```python
from build123d import *

# Parameters (mm, degrees)
SKETCH1_W             = 40
SKETCH1_H             = 51.5
BOSS_EXTRUDE1_DEPTH   = 18
SKETCH3_R             = 1.6
CUT_EXTRUDE1_DEPTH    = 19
SKETCH4_R             = 3.5
CUT_EXTRUDE2_DEPTH    = 18
CUT_EXTRUDE3_DEPTH    = 8
SKETCH6_R             = 9
CUT_EXTRUDE4_DEPTH    = 8
SKETCH7_R             = 7
CUT_EXTRUDE5_DEPTH    = 2.8
SKETCH8_R             = 6
CUT_EXTRUDE6_DEPTH    = 3.8
SKETCH9_R             = 5
CUT_EXTRUDE7_DEPTH    = 8
M3X0_5_TAPPED_HOLE1_D = 2.5
CUT_EXTRUDE8_DEPTH    = 2
CUT_EXTRUDE9_DEPTH    = 1
CHAMFER1_SIZE         = 0.8
SKETCH14_W            = 1
SKETCH14_H            = 6.5
CUT_EXTRUDE10_DEPTH   = 7


with BuildPart() as part:
    # Sketch1 → Boss-Extrude1 (new body)
    with BuildSketch(Plane.XY):
        Rectangle(SKETCH1_W, SKETCH1_H)
    extrude(amount=BOSS_EXTRUDE1_DEPTH)

    # Sketch3 → Cut-Extrude1 (cut, through all)
    with BuildSketch(Plane.XY.offset(18)):
        with Locations((-15, 21.5)):
            Circle(SKETCH3_R)
        with Locations((-15, -21.5)):
            Circle(SKETCH3_R)
        with Locations((15, 21.5)):
            Circle(SKETCH3_R)
        with Locations((15, -21.5)):
            Circle(SKETCH3_R)
    extrude(amount=-CUT_EXTRUDE1_DEPTH, mode=Mode.SUBTRACT)

    # Sketch4 → Cut-Extrude2 (cut)
    with BuildSketch(Plane.XY.offset(18)):
        with Locations((0, -14.25)):
            Circle(SKETCH4_R)
    extrude(amount=-CUT_EXTRUDE2_DEPTH, mode=Mode.SUBTRACT)

    # Sketch5 → Cut-Extrude3 (cut)
    with BuildSketch(Plane.XY.offset(18)):
        with BuildLine():
            Line((-17, 17.872848693), (-17, -17.872848693))
            ThreePointArc((-17, -17.872848693), (-17.124132538, -18.49783351), (-17.477686074, -19.027941805))
            ThreePointArc((-17.477686074, -19.027941805), (-17.229095042, -24.198357888), (-12.104699799, -23.466529111))
            ThreePointArc((-12.104699799, -23.466529111), (-11.517289712, -22.940191537), (-10.751842764, -22.75))
            Line((-10.751842764, -22.75), (-9.2376, -22.75))
            ThreePointArc((-9.2376, -22.75), (-8.237593216, -22.482046891), (-7.50554136, -21.749986433))
            Line((-7.50554136, -21.749986433), (-4.85642932, -17.161506784))
            ThreePointArc((-4.85642932, -17.161506784), (-4.082002001, -16.665704301), (-3.230119897, -17.011904614))
            ThreePointArc((-3.230119897, -17.011904614), (-3.134851007, -17.11961684), (-3.035950666, -17.224004614))
            ThreePointArc((-3.035950666, -17.224004614), (-2.824243732, -17.545979208), (-2.75, -17.9241))
            Line((-2.75, -17.9241), (-2.75, -20.75))
            ThreePointArc((-2.75, -20.75), (-2.164213562, -22.164213562), (-0.75, -22.75))
            Line((-0.75, -22.75), (10.751842764, -22.75))
            ThreePointArc((10.751842764, -22.75), (11.517289712, -22.940191537), (12.104699799, -23.466529111))
            ThreePointArc((12.104699799, -23.466529111), (17.229095042, -24.198357888), (17.477686074, -19.027941805))
            ThreePointArc((17.477686074, -19.027941805), (17.124132538, -18.49783351), (17, -17.872848693))
            Line((17, -17.872848693), (17, 17.872848693))
            ThreePointArc((17, 17.872848693), (17.124132538, 18.49783351), (17.477686074, 19.027941805))
            ThreePointArc((17.477686074, 19.027941805), (17.229095042, 24.198357888), (12.104699799, 23.466529111))
            ThreePointArc((12.104699799, 23.466529111), (11.517289712, 22.940191537), (10.751842764, 22.75))
            Line((10.751842764, 22.75), (-10.751842764, 22.75))
            ThreePointArc((-10.751842764, 22.75), (-11.517289712, 22.940191537), (-12.104699799, 23.466529111))
            ThreePointArc((-12.104699799, 23.466529111), (-17.229095042, 24.198357888), (-17.477686074, 19.027941805))
            ThreePointArc((-17.477686074, 19.027941805), (-17.124132538, 18.49783351), (-17, 17.872848693))
        make_face()
    extrude(amount=-CUT_EXTRUDE3_DEPTH, mode=Mode.SUBTRACT)

    # Sketch6 → Cut-Extrude4 (cut)
    with BuildSketch(Plane(origin=(0, 0, 0), x_dir=(-1, 0, 0), z_dir=(0, 0, -1))):
        with BuildLine():
            Line((-20, 10.5), (-15.5, 10.5))
            ThreePointArc((-15.5, 10.5), (-12.25, 7.25), (-15.5, 4))
            Line((-15.5, 4), (-20, 4))
            Line((-20, 4), (-20, -25.75))
            Line((-20, -25.75), (20, -25.75))
            Line((20, -25.75), (20, 4))
            Line((20, 4), (15.5, 4))
            ThreePointArc((15.5, 4), (12.25, 7.25), (15.5, 10.5))
            Line((15.5, 10.5), (20, 10.5))
            Line((20, 10.5), (20, 25.75))
            Line((20, 25.75), (-20, 25.75))
            Line((-20, 25.75), (-20, 10.5))
        make_face()
        with Locations((0, -14.25)):
            Circle(SKETCH6_R, mode=Mode.SUBTRACT)
    extrude(amount=-CUT_EXTRUDE4_DEPTH, mode=Mode.SUBTRACT)

    # Sketch7 → Cut-Extrude5 (cut)
    with BuildSketch(Plane(origin=(0, 0, 0), x_dir=(-1, 0, 0), z_dir=(0, 0, -1))):
        with Locations((0, -14.25)):
            Circle(SKETCH7_R)
    extrude(amount=-CUT_EXTRUDE5_DEPTH, mode=Mode.SUBTRACT)

    # Sketch8 → Cut-Extrude6 (cut)
    with BuildSketch(Plane(origin=(0, 0, 0), x_dir=(-1, 0, 0), z_dir=(0, 0, -1))):
        with Locations((0, -14.25)):
            Circle(SKETCH8_R)
    extrude(amount=-CUT_EXTRUDE6_DEPTH, mode=Mode.SUBTRACT)

    # Sketch9 → Cut-Extrude7 (cut)
    with BuildSketch(Plane(origin=(0, 0, 0), x_dir=(-1, 0, 0), z_dir=(0, 0, -1))):
        with Locations((0, -14.25)):
            Circle(SKETCH9_R)
    extrude(amount=-CUT_EXTRUDE7_DEPTH, mode=Mode.SUBTRACT)

    # M3x0.5 Tapped Hole1 (through all)
    with Locations(Plane(origin=(0, 0, 0), x_dir=(-1, 0, 0), z_dir=(0, 0, -1))):
        with Locations((-15.5, 7.25), (15.5, 7.25)):
            Hole(M3X0_5_TAPPED_HOLE1_D / 2)

    # Sketch12 → Cut-Extrude8 (cut)
    with BuildSketch(Plane(origin=(0, 0, 8), x_dir=(-1, 0, 0), z_dir=(0, 0, -1))):
        with BuildLine():
            Line((-8, 17.401970252), (-8, 25.75))
            Line((-8, 25.75), (8, 25.75))
            Line((8, 25.75), (8, 17.401970252))
            ThreePointArc((8, 17.401970252), (8.155139905, 16.629641806), (8.596491228, 15.977132322))
            ThreePointArc((8.596491228, 15.977132322), (0, -5), (-8.596491228, 15.977132322))
            ThreePointArc((-8.596491228, 15.977132322), (-8.155139905, 16.629641806), (-8, 17.401970252))
        make_face()
    extrude(amount=-CUT_EXTRUDE8_DEPTH, mode=Mode.SUBTRACT)

    # Sketch13 → Cut-Extrude9 (cut)
    with BuildSketch(Plane(origin=(0, 0, 0), x_dir=(-1, 0, 0), z_dir=(0, 0, -1))):
        with BuildLine():
            Line((-20, 10.5), (-20, 4))
            Line((-20, 4), (-15.5, 4))
            ThreePointArc((-15.5, 4), (-12.25, 7.25), (-15.5, 10.5))
            Line((-15.5, 10.5), (-20, 10.5))
        make_face()
        with BuildLine():
            Line((20, 4), (20, 10.5))
            Line((20, 10.5), (15.5, 10.5))
            ThreePointArc((15.5, 10.5), (12.25, 7.25), (15.5, 4))
            Line((15.5, 4), (20, 4))
        make_face()
    extrude(amount=-CUT_EXTRUDE9_DEPTH, mode=Mode.SUBTRACT)

    # Chamfer1
    chamfer1_edges = [part.edges().sort_by_distance(p)[0] for p in [
        (20, -25.75, 13),
        (-20, -25.75, 13),
        (-20, 25.75, 13),
        (20, 25.75, 13),
    ]]
    chamfer(chamfer1_edges, length=CHAMFER1_SIZE)

    # Sketch14 → Cut-Extrude10 (cut)
    with BuildSketch(Plane(origin=(0, 0, 1), x_dir=(-1, 0, 0), z_dir=(0, 0, -1))):
        with Locations((-19.5, 7.25)):
            Rectangle(SKETCH14_W, SKETCH14_H)
        with Locations((19.5, 7.25)):
            Rectangle(SKETCH14_W, SKETCH14_H)
    extrude(amount=-CUT_EXTRUDE10_DEPTH, mode=Mode.SUBTRACT)


solid = part.part
```
Model file for the job. Use its own axes, mm. A direction names the side the tool comes from. Round coordinates to 2 decimals unless told otherwise and drop trailing zeros. Order: outer loops, then holes, each group sorted by start corner. A loop starts at its lowest first (then second) coordinate and runs counter-clockwise, first axis right, second up. Notation, with made-up numbers: (-1.5, 9) -> (40.5, 9) arc R20 ccw to (40.5, 14) -> close; hole circle Ø4 at (9.5, 82.25). An arc over 180 degrees is marked (long way). Use one line per item in the form item = value.
Item 1: Drill centre lines: line 1 (X direction, y = -10.5, z = 14); line 2 (Y direction, x = 8, z = 14.5); line 3 (Y direction, x = -15, z = 9.4). Where is each one in solid material? Low to high.
Returned:
line_1 = -20 to -17, 17 to 20
line_2 = -25.75 to -22.75, 22.75 to 25.75
line_3 = -25.75 to -23.1, -19.9 to 6.1, 8.4 to 19.9, 23.1 to 25.75
Item 2: Cut at B-B, the plane z = 4.75. Write the cut outline in (x, y), and give its area (3 significant figures).
Returned:
outline = (-19, 4) -> (-15.5, 4) arc R3.25 ccw to (-15.5, 10.5) -> (-19, 10.5) -> close; circle Ø18 at (0, -14.25); (15.5, 4) -> (19, 4) -> (19, 10.5) -> (15.5, 10.5) arc R3.25 ccw to start; hole circle Ø2.5 at (-15.5, 7.25); hole circle Ø10 at (0, -14.25); hole circle Ø2.5 at (15.5, 7.25)
area = 245 mm^2
Item 3: Cut at C-C, the plane x = 0. Give the number of separate pieces and of enclosed holes in the cut face, and give its area (3 significant figures).
Returned:
separate_pieces = 3
enclosed_holes = 0
area = 126 mm^2
Item 4: Flat gauge pins, fed straight in: pin 1 Ø3.5 at (x, y) = (15, 21.5) entering from -Z; pin 2 Ø2 at (y, z) = (10.5, 4.5) entering from +X; pin 3 Ø2 at (x, y) = (15.5, 8.5) entering from -Z. Where does each tip first touch, or does it go through?
Returned:
pin_1 = 8
pin_2 = 19
pin_3 = 1
Item 5: Tool access for faces 1 (the face through (-8.15, 16.64, 8.99)), 2 (the face through (-17, 4, 4)), 3 (the face through (17.166, -24.25, 14.056)), 4 (the face through (-6, -12, 2.8)): list every direction of +Z, -Z, +X, -X, +Y, -Y with a clear straight run to the whole face (end or side of a thin tool).
Returned:
face_1 = +Z, -Z
face_2 = -Z, +X, -X, -Y
face_3 = +Z
face_4 = -Z
Item 6: Pull direction X, two halves, no side cores. Call faces 5 (the face through (20, 0, 13)), 6 (the face through (0, -25.75, 13)), 7 (the face through (-6.2, -19.49, 14.06)), 8 (the face through (-19, 7, 4)): released by +X, released by -X, zero draft, split by the parting line, or undercut.
Returned:
face_5 = released by +X
face_6 = zero draft
face_7 = undercut
face_8 = released by -X
Item 7: Cut at A-A, the plane y = 21.5. Write the cut outline in (x, z).
Returned:
outline = (-20, 8) -> (-16.6, 8) -> (-16.6, 10) -> (-18.5, 10) -> (-18.5, 18) -> (-20, 18) -> close; (-13.4, 8) -> (-8, 8) -> (-8, 10) -> (-13.4, 10) -> close; (8, 8) -> (13.4, 8) -> (13.4, 10) -> (8, 10) -> close; (16.6, 8) -> (20, 8) -> (20, 18) -> (18.5, 18) -> (18.5, 10) -> (16.6, 10) -> close
